from build123d import *

# Parameters (mm, degrees)
SKETCH_2_W      = 120
SKETCH_2_H      = 20
SKETCH_2_R      = 2.5
SKETCH_2_R_2    = 4
EXTRUDE_1_DEPTH = 2


with BuildPart() as part:
    # Эскиз2 → Бобышка-Вытянуть1 (new body)
    with BuildSketch(Plane(origin=(0, 0, 0), x_dir=(1, 0, 0), z_dir=(0, 1, 0))):
        Rectangle(SKETCH_2_W, SKETCH_2_H)
        with Locations(Location((-50, 5, 0), (0, 0, 270))):
            Circle(SKETCH_2_R, mode=Mode.SUBTRACT)
        with Locations(Location((-10, 5, 0), (0, 0, 270))):
            Circle(SKETCH_2_R, mode=Mode.SUBTRACT)
        with Locations(Location((30, 5, 0), (0, 0, 270))):
            Circle(SKETCH_2_R, mode=Mode.SUBTRACT)
        with Locations(Location((-30, -5, 0), (0, 0, 270))):
            Circle(SKETCH_2_R, mode=Mode.SUBTRACT)
        with Locations(Location((10, -5, 0), (0, 0, 270))):
            Circle(SKETCH_2_R, mode=Mode.SUBTRACT)
        with Locations(Location((50, -5, 0), (0, 0, 270))):
            Circle(SKETCH_2_R, mode=Mode.SUBTRACT)
        with Locations(Location((-40, 0, 0), (0, 0, 270))):
            Circle(SKETCH_2_R_2, mode=Mode.SUBTRACT)
        with Locations(Location((15, 0, 0), (0, 0, 270))):
            Circle(SKETCH_2_R_2, mode=Mode.SUBTRACT)
    extrude(amount=EXTRUDE_1_DEPTH)


solid = part.part
Design review of the part built by this model. Coordinates are the model's own, in mm. Coordinates: 2 decimals unless noted, no trailing zeros. Loops run counter-clockwise (first coordinate to the right, second up) from the corner with the lowest first, then second, coordinate; pieces in that order, holes last. Notation, with made-up numbers: (33.5, 22) -> (64.5, 22) arc R10 ccw to (64.5, 32) -> close; hole circle Ø3 at (84, 39). An arc over 180 degrees is marked (long way). Use a Markdown table: item, result. Add a question column.
Item 1: We need section A-A, the plane y = 0.65. Count the separate pieces of the cut face and the enclosed holes in it, and give its area (3 significant figures).
Item 2: We need section B-B, the plane x = -40. Write out the cut boundary in (y, z), and give its area (3 significant figures).
Item 3: We need section D-D, the plane x = 50. Write out the cut boundary in (y, z).
Item 4: Clearance check with a flat-ended pin moving along its axis: P1, Ø6.5, axis at x = 10, z = 5, coming from the +Y side. State where the tip first meets the part, or that it passes through.
Item 5: Wall thickness on L1, parallel to X at y = 1.4, z = -5; L2, parallel to X at y = 1.45, z = 5; L3, parallel to X at y = 0.9, z = 0: over which ranges is each line inside the solid? List them lowest first. Write a range as from..to.
Item 6: We need section C-C, the plane z = 0. Write out the cut boundary in (x, y).
Item 7: The part is to be moulded in two halves that separate along X. For faces 1 (the flat face through (-1, 0, 0)), 2 (the cylindrical face through (-27.89, 0.99, 6.34)), 3 (the flat face through (-60, 1, 0)), say which applies: +X half, -X half, draft (parallel to the pull), parting line (faces both ways), or undercut.
Numbers:
| question | item | result |
|---|---|---|
| 1 | separate pieces | 1 |
| 1 | enclosed holes | 8 |
| 1 | area | 2,180 mm^2 |
| 2 | outline | (0, -10) -> (2, -10) -> (2, -4) -> (0, -4) -> close; (0, 4) -> (2, 4) -> (2, 10) -> (0, 10) -> close |
| 2 | area | 24.0 mm^2 |
| 3 | outline | (0, -10) -> (2, -10) -> (2, 2.5) -> (0, 2.5) -> close; (0, 7.5) -> (2, 7.5) -> (2, 10) -> (0, 10) -> close |
| 4 | P1 | stops at y = 2 |
| 5 | L1 | x = -60..-52.5, -47.5..-12.5, -7.5..27.5, 32.5..60 |
| 5 | L2 | x = -60..-32.5, -27.5..7.5, 12.5..47.5, 52.5..60 |
| 5 | L3 | x = -60..-44, -36..11, 19..60 |
| 6 | outline | (-60, 0) -> (-44, 0) -> (-44, 2) -> (-60, 2) -> close; (-36, 0) -> (11, 0) -> (11, 2) -> (-36, 2) -> close; (19, 0) -> (60, 0) -> (60, 2) -> (19, 2) -> close |
| 7 | face 1 | draft |
| 7 | face 2 | undercut |
| 7 | face 3 | -X half |
